Could you check a few things on this model? Use its own coordinates, in mm. Give positions to 0.01 mm unless a question says otherwise; leave off trailing zeros. Loops run counter-clockwise (first coordinate to the right, second up) from the corner with the lowest first, then second, coordinate; pieces in that order, holes last. Notation, with made-up numbers: (-16, 2) - (26, 2) arc R21 cw to (26, 38) - close; hole circle Ø3 at (62, 33). An arc over 180 degrees is marked (long way). Write each question's results on one line, items separated by ' | '. Start each with the question number.
(1) For pin 1 (6 mm diameter, centred on x = 35.75, y = 0, fed in from +Z), with a flat end and sliding along its axis, tell me the tip position at first contact or that it passes through.
(2) Suppose I cut it at A-A (x = 10). Please give me the cut outline in (y, z).
(3) I need wall thicknesses on line 1 (Y direction, x = 11, z = 0.35); line 2 (Y direction, x = -35.75, z = 1.75); line 3 (X direction, y = -1, z = 2.95). Which ranges of each line are inside material? Lowest first, please.
(4) Suppose I cut it at C-C (z = 0.8). Please give me the cut outline in (x, y).
(5) Suppose I cut it at B-B (y = 0). Please give me the cut outline in (x, z).
from build123d import *

# Parameters (mm, degrees)
SKETCH_R        = 5
PAD_DEPTH       = 4
CHAMFER_SIZE    = 1
CHAMFER001_SIZE = 1
CHAMFER002_SIZE = 1


with BuildPart() as part:
    # Sketch → Pad (new body)
    with BuildSketch(Plane.XY):
        with BuildLine():
            ThreePointArc((-35.75, 15), (-50.75, 0), (-35.75, -15))
            Line((-35.75, -15), (35.75, -15))
            ThreePointArc((35.75, -15), (50.75, 0), (35.75, 15))
            Line((-35.75, 15), (35.75, 15))
        make_face()
        with Locations((-35.75, 0)):
            Circle(SKETCH_R, mode=Mode.SUBTRACT)
        with Locations((35.75, 0)):
            Circle(SKETCH_R, mode=Mode.SUBTRACT)
        with BuildLine():
            ThreePointArc((-11.85289, 9), (-20.85289, 0), (-11.85289, -9))
            Line((-11.85289, -9), (11.85289, -9))
            ThreePointArc((11.85289, -9), (20.85289, 0), (11.85289, 9))
            Line((-11.85289, 9), (11.85289, 9))
        make_face(mode=Mode.SUBTRACT)
    extrude(amount=PAD_DEPTH)

    # Chamfer
    chamfer_edges = [part.edges().sort_by_distance(p)[0] for p in [
        (-40.75, 0, 4),
        (30.75, 0, 4),
    ]]
    chamfer(chamfer_edges, length=CHAMFER_SIZE)

    # Chamfer001
    chamfer001_edges = [part.edges().sort_by_distance(p)[0] for p in [
        (0, 15, 4),
        (50.75, 0, 4),
        (0, -15, 4),
        (-50.75, 0, 4),
    ]]
    chamfer(chamfer001_edges, length=CHAMFER001_SIZE)

    # Chamfer002
    chamfer002_edges = [part.edges().sort_by_distance(p)[0] for p in [
        (20.85289, 0, 4),
        (0, -9, 4),
        (-20.85289, 0, 4),
        (0, 9, 4),
    ]]
    chamfer(chamfer002_edges, length=CHAMFER002_SIZE)


solid = part.part
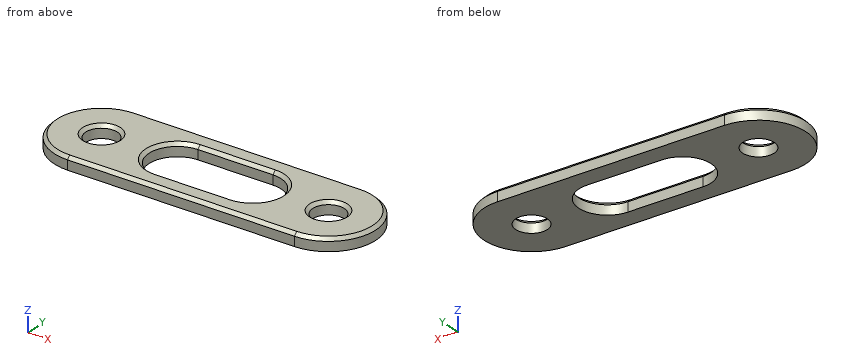
Output values:
1) pin 1: through
2) outline: (-15, 0) - (-9, 0) - (-9, 3) - (-10, 4) - (-14, 4) - (-15, 3) - close; (9, 0) - (15, 0) - (15, 3) - (14, 4) - (10, 4) - (9, 3) - close
3) line 1: -15 to -9, 9 to 15 | line 2: -15 to -5, 5 to 15 | line 3: -50.72 to -40.65, -30.85 to -20.8, 20.8 to 30.85, 40.65 to 50.72
4) outline: (-35.75, -15) - (35.75, -15) arc R15 ccw to (35.75, 15) - (-35.75, 15) arc R15 ccw to start; hole circle Ø10 at (-35.75, 0); hole (-11.85, -9) - (11.85, -9) arc R9 ccw to (11.85, 9) - (-11.85, 9) arc R9 ccw to start; hole circle Ø10 at (35.75, 0)
5) outline: (-50.75, 0) - (-40.75, 0) - (-40.75, 3) - (-41.75, 4) - (-49.75, 4) - (-50.75, 3) - close; (-30.75, 0) - (-20.85, 0) - (-20.85, 3) - (-21.85, 4) - (-29.75, 4) - (-30.75, 3) - close; (20.85, 0) - (30.75, 0) - (30.75, 3) - (29.75, 4) - (21.85, 4) - (20.85, 3) - close; (40.75, 0) - (50.75, 0) - (50.75, 3) - (49.75, 4) - (41.75, 4) - (40.75, 3) - close
